```python
from build123d import *

# Parameters (mm, degrees)
SKETCH1_R           = 7.5
BOSS_EXTRUDE1_DEPTH = 102
SKETCH2_R           = 5
BOSS_EXTRUDE2_DEPTH = 1
SKETCH3_R           = 4
BOSS_EXTRUDE3_DEPTH = 29
SKETCH4_R           = 3.5
BOSS_EXTRUDE4_DEPTH = 1
SKETCH5_R           = 2.5
BOSS_EXTRUDE5_DEPTH = 5


with BuildPart() as part:
    # Sketch1 → Boss-Extrude1 (new body)
    with BuildSketch(Plane(origin=(0, 0, 0), x_dir=(1, 0, 0), z_dir=(0, 1, 0))):
        with Locations(Location((0, 0, 0), (0, 0, 270))):
            Circle(SKETCH1_R)
    extrude(amount=BOSS_EXTRUDE1_DEPTH)

    # Sketch2 → Boss-Extrude2 (add)
    with BuildSketch(Plane.XZ):
        with Locations(Location((0, 0, 0), (0, 0, 270))):
            Circle(SKETCH2_R)
    extrude(amount=BOSS_EXTRUDE2_DEPTH)

    # Sketch3 → Boss-Extrude3 (add)
    with BuildSketch(Plane.XZ.offset(1)):
        with Locations(Location((0, 0, 0), (0, 0, 90))):
            Circle(SKETCH3_R)
    extrude(amount=BOSS_EXTRUDE3_DEPTH)

    # Sketch4 → Boss-Extrude4 (add)
    with BuildSketch(Plane(origin=(0, 102, 0), x_dir=(1, 0, 0), z_dir=(0, 1, 0))):
        with Locations(Location((0, 0, 0), (0, 0, 270))):
            Circle(SKETCH4_R)
    extrude(amount=BOSS_EXTRUDE4_DEPTH)

    # Sketch5 → Boss-Extrude5 (add)
    with BuildSketch(Plane(origin=(0, 103, 0), x_dir=(1, 0, 0), z_dir=(0, 1, 0))):
        with Locations(Location((0, 0, 0), (0, 0, 270))):
            Circle(SKETCH5_R)
    extrude(amount=BOSS_EXTRUDE5_DEPTH)


solid = part.part
```
CAD build for the part. Positions are in the model's coordinates, mm. A direction names the side the tool comes from. Coordinates: 2 decimals unless noted, no trailing zeros. Write each loop counter-clockwise with the first axis right and the second up, starting at its lowest first coordinate (ties: lowest second). Pieces come first, ordered by that corner, then holes.
(1) Cut at C-C, the plane y = 17. List the corners of the cut face in (x, z), and give its area (3 significant figures).
(2) 3-axis set-ups, long thin cutter, end or side, ignore diameter. For faces 1 (the face through (-2.44, 105.46, -0.54)), 2 (the face through (0, 108, 0)), 3 (the face through (3.905, -15.297, -0.867)): which of +Z, -Z, +X, -X, +Y, -Y reach the whole face in a straight line?
(3) Drill centre lines: probe 1 along X at (y, z) = (37.5, 0.25); probe 2 along Y at (x, z) = (-5.25, -5); probe 3 along Y at (x, z) = (2.5, -4). Where is each one in solid material? Low to high.
(4) Flat gauge pins, fed straight in: pin 1 (5 mm diameter, centred on y = -16, z = 1.5, fed in from -X); pin 2 (2 mm diameter, centred on x = 2.5, y = 91, fed in from -Z); pin 3 (4 mm diameter, centred on y = 50.5, z = 4, fed in from +X). Where does each tip first touch, or does it go through?
(5) Cut at A-A, the plane x = 0. List the corners of the cut face in (y, z), and give its area (3 significant figures).
(6) Cut at B-B, the plane z = 0. List the corners of the cut face in (x, y).
Geometry says:
1. outline: circle Ø15 at (0, 0)
1. area: 177 mm2
2. face 1: +Y
2. face 2: +Z, -Z, +X, -X, +Y
2. face 3: -Y
3. probe 1: x = -7.5 to 7.5
3. probe 2: y = 0 to 102
3. probe 3: y = -1 to 102
4. pin 1: stops at x = -4
4. pin 2: stops at z = -7.35
4. pin 3: stops at x = 7.23
5. outline: (-30, -4) - (-1, -4) - (-1, -5) - (0, -5) - (0, -7.5) - (102, -7.5) - (102, -3.5) - (103, -3.5) - (103, -2.5) - (108, -2.5) - (108, 2.5) - (103, 2.5) - (103, 3.5) - (102, 3.5) - (102, 7.5) - (0, 7.5) - (0, 5) - (-1, 5) - (-1, 4) - (-30, 4) - close
5. area: 1,800 mm2
6. outline: (-7.5, 0) - (-5, 0) - (-5, -1) - (-4, -1) - (-4, -30) - (4, -30) - (4, -1) - (5, -1) - (5, 0) - (7.5, 0) - (7.5, 102) - (3.5, 102) - (3.5, 103) - (2.5, 103) - (2.5, 108) - (-2.5, 108) - (-2.5, 103) - (-3.5, 103) - (-3.5, 102) - (-7.5, 102) - close
